from build123d import *

# Parameters (mm, degrees)
SKETCH_1_W                    = 3.75
SKETCH_1_H                    = 0.7
REVOLVE_1_ANGLE               = 30
EXTRUDE_1_DEPTH               = 1.5
EXTRUDE_START                 = -4.1
SKETCH_3_R                    = 21.25
EXTRUDE_2_DEPTH               = 4.1
HOLE_WIZARD_2_5_2_5_1_D       = 2.5
HOLE_WIZARD_17_5_17_5_1_D     = 17.5
HOLE_WIZARD_17_5_17_5_1_DEPTH = 6.3
HOLE_WIZARD_M3_1_D            = 3.4
HOLE_WIZARD_M3_1_DEPTH        = 6.3
HOLE_WIZARD_M3_1_CBORE_D      = 6.5
HOLE_WIZARD_M3_1_CBORE_DEPTH  = 3.5
FILLET_1_R                    = 0.5
FILLET_2_R                    = 1


with BuildPart() as part:
    # 草图1 → 旋转1 (revolve)
    with BuildSketch(Plane(origin=(0, 0, 0), x_dir=(0.34202014332566955, 0.9396926207859082, 0), z_dir=(0.9396926207859082, -0.34202014332566955, 0))):
        with Locations((19.375, -0.35)):
            Rectangle(SKETCH_1_W, SKETCH_1_H)
    revolve(axis=Axis((0, 0, 0), (0, 0, 1)), revolution_arc=REVOLVE_1_ANGLE)

    # 草图2 → 凸台-拉伸1 (add)
    with BuildSketch(Plane.XY):
        with BuildLine():
            Line((-3.038843109, 17.234135678), (-3.690023775, 20.927164752))
            ThreePointArc((-3.690023775, 20.927164752), (1.852059533, 21.169137334), (7.267928046, 19.968468192))
            Line((7.267928046, 19.968468192), (5.985352508, 16.444620864))
            ThreePointArc((5.985352508, 16.444620864), (6.73975713, 14.511225787), (8.703707451, 15.18207748))
            ThreePointArc((8.703707451, 15.18207748), (-1.525225498, -17.433407217), (-5.93513849, 16.462810547))
            ThreePointArc((-5.93513849, 16.462810547), (-4.117517161, 15.461114204), (-3.038843109, 17.234135678))
        make_face()
    extrude(amount=EXTRUDE_1_DEPTH)

    # 草图3 → 凸台-拉伸2 (add)
    with BuildSketch(Plane(origin=(0, 0, 1.5), x_dir=(-1, 0, 0), z_dir=(0, 0, -1)).offset(EXTRUDE_START)):
        with Locations(Location((0, 0, 0), (0, 0, 80))):
            Circle(SKETCH_3_R)
    extrude(amount=EXTRUDE_2_DEPTH)

    # Ø2.5 (2.5) 直径孔1 (through all)
    with Locations(Plane(origin=(0, 0, 0), x_dir=(-1, 0, 0), z_dir=(0, 0, -1))):
        with Locations((13.448628424, 1.176602527), (7.743281891, -11.058552598), (-5.705346534, -12.235155125), (-13.448628424, -1.176602527), (-7.743281891, 11.058552598), (5.705346533, 12.235155125)):
            Hole(HOLE_WIZARD_2_5_2_5_1_D / 2)

    # Ø17.5 (17.5) 直径孔1
    with Locations(Plane.XY.offset(5.6)):
        with Locations((0, 0)):
            Hole(HOLE_WIZARD_17_5_17_5_1_D / 2, depth=HOLE_WIZARD_17_5_17_5_1_DEPTH)

    # M3 六角头机械螺钉的柱形沉头孔1
    with Locations(Plane.XY.offset(5.6)):
        with Locations((12.235155125, 5.705346533), (1.176602527, 13.448628424), (-11.058552598, 7.743281891), (-12.235155125, -5.705346533), (-1.176602527, -13.448628424), (11.058552598, -7.743281891)):
            CounterBoreHole(HOLE_WIZARD_M3_1_D / 2, HOLE_WIZARD_M3_1_CBORE_D / 2, HOLE_WIZARD_M3_1_CBORE_DEPTH, depth=HOLE_WIZARD_M3_1_DEPTH)

    # 圆角1
    # the kernel refuses this fillet: 0.5 mm, written as the material it takes off along each edge
    with BuildSketch(Plane(origin=(-3.038843109, 17.234135678, 0), x_dir=(-0.17364817766693064, 0.984807753012208, -5.075305255429288e-15), z_dir=(0, 0, -1))) as fillet_1_piece_1:
        with BuildLine():
            CenterArc((0.493054215, 0.5), FILLET_1_R, 181.591754177, 88.408245823)
            ThreePointArc((-0.006752846, 0.486111111), (-0.001688293, 0.243079006), (0, 0))
            Line((0, 0), (0.493054215, 0))
        make_face()
    extrude(amount=1.932635539, mode=Mode.SUBTRACT)
    with BuildSketch(Plane(origin=(5.985352508, 16.444620864, 0), x_dir=(0.34202014332566866, 0.9396926207859084, -5.075305255429287e-15), z_dir=(0, 0, -1))) as fillet_1_piece_2:
        with BuildLine():
            CenterArc((0.493054215, -0.5), FILLET_1_R, 90, 88.408245823)
            ThreePointArc((-0.006752846, -0.486111111), (-0.001688293, -0.243079006), (0, 0))
            Line((0, 0), (0.493054215, 0))
        make_face()
    extrude(amount=1.932635539, mode=Mode.SUBTRACT)
    with BuildSketch(Plane(origin=(7.267928046, 19.968468192, 1.5), x_dir=(-0.943745429784676, 0.33067289541257716, 0), z_dir=(0, 0, -1)), Plane(origin=(-3.690023775, 20.927164752, -1.980213416), x_dir=(0.9868285618140304, 0.1617695570496889, 5.378398972447093e-15), z_dir=(0, 0, 1))) as fillet_1_piece_3:
        with BuildLine():
            CenterArc((0.506060833, -0.499963704), FILLET_1_R, 89.309622583, 91.380754834)
            Line((0.006097129, -0.505988237), (0, 0))
            ThreePointArc((0, 0), (0.256042683, 0.001542594), (0.512085366, 0))
        make_face()
    extrude(amount=3.480213416, mode=Mode.SUBTRACT)
    with BuildSketch(Plane(origin=(5.985352508, 16.444620864, 0), x_dir=(0.3420201433260408, 0.9396926207857731, 0), z_dir=(0, 0, 1))) as fillet_1_piece_4:
        with BuildLine():
            CenterArc((0.009949299, 0.5), FILLET_1_R, 267.872834894, 2.127165106)
            ThreePointArc((-0.008609454, 0.000344546), (-0.00430448, 0.000178455), (0, 0))
            Line((0, 0), (0.009949299, 0))
        make_face()
    extrude(amount=1.5, mode=Mode.SUBTRACT)
    with BuildSketch(Plane(origin=(-3.038843109, 17.234135678, 0), x_dir=(-0.17364817766558338, 0.9848077530124456, 0), z_dir=(0, 0, 1))) as fillet_1_piece_5:
        with BuildLine():
            CenterArc((0.009949299, -0.5), FILLET_1_R, 90, 2.127165106)
            ThreePointArc((-0.008609454, -0.000344546), (-0.00430448, -0.000178455), (0, 0))
            Line((0, 0), (0.009949299, 0))
        make_face()
    extrude(amount=1.5, mode=Mode.SUBTRACT)

    # 圆角2
    fillet_2_edges = [part.edges().sort_by_distance(p)[0] for p in [
        (-5.93513849, 16.462810547, 0.75),
        (8.703707451, 15.18207748, 0.75),
    ]]
    fillet(fillet_2_edges, radius=FILLET_2_R)


solid = part.part
Source: CAD feature listing. Evaluate the final solid. Frame: model axes, mm. A direction names the side the tool comes from. Round coordinates to 2 decimals unless told otherwise and drop trailing zeros. Order: outer loops, then holes, each group sorted by start corner. A loop starts at its lowest first (then second) coordinate and runs counter-clockwise, first axis right, second up. Notation, with made-up numbers: (77, 25) - (94, 25) arc R26 cw to (94, 58) - close; hole circle Ø7 at (-21.75, 88.25). An arc over 180 degrees is marked (long way). Use a Markdown table: item, result. Add a question column.
1. Line query: probe 1 along Y at (x, z) = (7, 1.75); probe 2 along Y at (x, z) = (-8, 1.25); probe 3 along X at (y, z) = (5, 0.75). Output: solid intervals per line, ascending.
2. Mould query, pull axis Y, two halves, no side actions, for faces 1 (the flat face through (8, -4, 0)), 2 (the cylindrical face through (-10.74, -8.59, 3.87)). Classes: +Y half, -Y half, draft (parallel to the pull), parting line (faces both ways), or undercut.
3. Set-up query: faces 3 (the flat face through (0, -18, 1.5)), 4 (the cylindrical face through (-13.857, -5.195, 1.035)), 5 (the cylindrical face through (-1.88, -16.62, 3.87)). Return all of +Z, -Z, +X, -X, +Y, -Y with unobstructed straight access to the full face (end or side cutting, diameter ignored); none if empty.
4. Section query A-A (z = 4). Give the number of separate pieces and of enclosed holes in the cut face, then the cut area to 3 significant figures.
5. First-contact query: pin 1 (2 mm diameter, centred on x = 16, z = 2.5, fed in from +Y); pin 2 (8 mm diameter, centred on x = 8.5, y = 11, fed in from -Z); pin 3 (4 mm diameter, centred on x = 12.24, y = 5.71, fed in from +Z). Flat tips, straight axial feed; report the tip coordinate or a pass-through.
6. Section query C-C (x = 0). Return the cut outline in (y, z), then the cut area to 3 significant figures.
7. Section query B-B (y = 5). Return the cut outline in (x, z), then the cut area to 3 significant figures.
Derived:
| question | item | result |
|---|---|---|
| 1 | probe 1 | -20.06 to -5.25, 5.25 to 10.05, 12.06 to 20.06 |
| 1 | probe 2 | -15.56 to -12.28, -9.84 to -3.54, 3.54 to 15.56 |
| 1 | probe 3 | -16.77 to -7.18, 7.18 to 10.69, 13.78 to 16.77 |
| 2 | face 1 | draft |
| 2 | face 2 | undercut |
| 3 | face 3 | -Z |
| 3 | face 4 | +Z, -Z |
| 3 | face 5 | +Z |
| 4 | separate pieces | 1 |
| 4 | enclosed holes | 13 |
| 4 | area | 950 mm2 |
| 5 | pin 1 | y = 15.05 |
| 5 | pin 2 | z = 0 |
| 5 | pin 3 | z = 2.1 |
| 6 | outline | (-21.25, 1.5) - (-17.5, 1.5) - (-17.5, 0) - (-14.68, 0) - (-14.68, 2.1) - (-16.48, 2.1) - (-16.48, 5.6) - (-21.25, 5.6) - close; (-12.22, 0) - (-8.75, 0) - (-8.75, 5.6) - (-10.42, 5.6) - (-10.42, 2.1) - (-12.22, 2.1) - close; (8.75, 0) - (12.22, 0) - (12.22, 2.1) - (10.42, 2.1) - (10.42, 5.6) - (8.75, 5.6) - close; (14.68, 0) - (17.5, 0) - (17.5, -0.7) - (21.25, -0.7) - (21.25, 5.6) - (16.48, 5.6) - (16.48, 2.1) - (14.68, 2.1) - close |
| 6 | area | 84.3 mm2 |
| 7 | outline | (-20.65, 1.5) - (-16.77, 1.5) - (-16.77, 0) - (-7.18, 0) - (-7.18, 5.6) - (-9.32, 5.6) - (-9.32, 2.1) - (-12.8, 2.1) - (-12.8, 5.6) - (-20.65, 5.6) - close; (7.18, 0) - (10.69, 0) - (10.69, 2.1) - (9.06, 2.1) - (9.06, 5.6) - (7.18, 5.6) - close; (13.78, 0) - (16.77, 0) - (16.77, 1.5) - (20.65, 1.5) - (20.65, 5.6) - (15.41, 5.6) - (15.41, 2.1) - (13.78, 2.1) - close |
| 7 | area | 98.3 mm2 |
